The model under review builds one solid part; all positions refer to its coordinate system, in mm. Face numbers are marked on the shaded views. A direction names the side the tool comes from. Round coordinates to 2 decimals unless told otherwise and drop trailing zeros. Order: outer loops, then holes, each group sorted by start corner. A loop starts at its lowest first (then second) coordinate and runs counter-clockwise, first axis right, second up. Notation, with made-up numbers: M 39.5,-10 L 58.5,-10 A10 cw 58.5,3 Z; hole C 36,52.5 d7. An arc over 180 degrees is marked long. Answer as a JSON object with one key per item and string values. Group by question number.
1) Consider section A-A, the plane y = 19. Write out the cut boundary in (x, z).
2) Insertion check: pin 1 Ø2 at (y, z) = (11.5, -5.5) entering from +X; pin 2 Ø3 at (x, z) = (36.75, -17.5) entering from +Y. Each pin has a flat end and moves straight along its axis. Give the tip position at first contact, or say it passes through.
3) To check wall thickness, follow line 1 (X direction, y = 1.4, z = -17.5); line 2 (X direction, y = 8, z = -12); line 3 (Y direction, x = 44.45, z = -30). State the ranges of each line that lie inside material, in increasing order.
4) For the marked faces 4 and 5, list the 3-axis set-ups (+Z, -Z, +X, -X, +Y, -Y) from which the entire face can be reached by the end or side of a thin tool; tool diameter is ignored.
5) The part is to be moulded in two halves that separate along X. For the marked faces 1, 2 and 3, say which applies: +X half, -X half, draft (parallel to the pull), parting line (faces both ways), or undercut.
6) Consider section D-D, the plane z = -17.5. Write out the cut boundary in (x, y).
7) Consider section C-C, the plane x = 9.25. Write out the cut boundary in (y, z), then the cut area to 3 significant figures.
8) Consider section B-B, the plane z = -21.5. Write out the cut boundary in (x, y).
Autodesk Inventor part; units mm, degrees
ref_plane "YZ Plane" through (0, 0, 0) normal (1, 0, 0) x (0, 1, 0)
ref_plane "XZ Plane" through (0, 0, 0) normal (0, 1, 0) x (-1, 0, 0)
ref_plane "XY Plane" through (0, 0, 0) normal (0, 0, 1) x (1, 0, 0)
sketch "Boceto1" plane through (0, 0, 0) normal (0, 0, 1) x (1, 0, 0)
  line L0 (0, 0) -> (46, 0)
  line L1 (46, 0) -> (46, 21)
  line L2 (46, 21) -> (43, 21)
  line L3 (43, 21) -> (43, 3)
  line L4 (43, 3) -> (3, 3)
  line L5 (3, 3) -> (3, 21)
  line L6 (3, 21) -> (0, 21)
  line L7 (0, 21) -> (0, 0)
extrude "Extrusión1" add sketch "Boceto1" against normal blind 35
sketch "Boceto2" plane through (46, 0, 0) normal (1, 0, 0) x (0, 0, -1)
  circle A0 centre (5, 12) radius 2.5
  circle A1 centre (30, 12) radius 2.5
extrude "Extrusión2" cut sketch "Boceto2" against normal blind 60 contours A0
extrude "Extrusión3" cut sketch "Boceto2" against normal blind 60 contours A1
fillet "Empalme1" radius 5 4 edges at (1.5, 21, 0) (1.5, 21, -35) (44.5, 21, 0) (44.5, 21, -35)
sketch "Boceto3" plane through (3, 3, 0) normal (0, 1, 0) x (1, 0, 0)
  line L0 (8.75, 23.5) -> (31.25, 23.5)
  line L1 (31.25, 23.5) -> (31.25, 11.5)
  line L2 (31.25, 11.5) -> (8.75, 11.5)
  line L3 (8.75, 11.5) -> (8.75, 23.5)
  line L4 (8.75, 23.5) -> (8.75, 17.5)
  circle A0 centre (6.25, 17.5) radius 1.25
  line L5 (31.25, 23.5) -> (31.25, 17.5)
  circle A1 centre (33.75, 17.5) radius 1.25
  point P0 (-3, 0)
  point P1 (0, 35)
extrude "Extrusión4" cut sketch "Boceto3" against normal blind 60 contours L0 L1 L2 L3
extrude "Extrusión5" cut sketch "Boceto3" against normal blind 60 contours A0 | A1
properties part number "8_1"
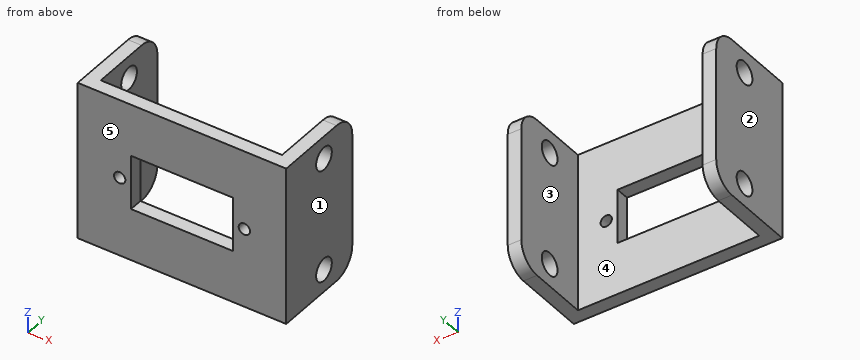
Results list:
{
 "1": {"outline": "M 0,-34 L 3,-34 L 3,-1 L 0,-1 Z; M 43,-34 L 46,-34 L 46,-1 L 43,-1 Z"},
 "2": {"pin 1": "through", "pin 2": "y = 3"},
 "3": {"line 1": "0 to 8, 10.5 to 11.75, 34.25 to 35.5, 38 to 46", "line 2": "0 to 3, 43 to 46", "line 3": "0 to 9.5, 14.5 to 21"},
 "4": {"face 4": "+Z, -Z, +Y", "face 5": "+Z, -Z, +X, -X, -Y"},
 "5": {"face 1": "+X half", "face 2": "-X half", "face 3": "undercut"},
 "6": {"outline": "M 0,0 L 8,0 L 8,3 L 3,3 L 3,21 L 0,21 Z; M 10.5,0 L 11.75,0 L 11.75,3 L 10.5,3 Z; M 34.25,0 L 35.5,0 L 35.5,3 L 34.25,3 Z; M 38,0 L 46,0 L 46,21 L 43,21 L 43,3 L 38,3 Z"},
 "7": {"outline": "M 0,-35 L 3,-35 L 3,-18.75 L 0,-18.75 Z; M 0,-16.25 L 3,-16.25 L 3,0 L 0,0 Z", "area": "97.5 mm^2"},
 "8": {"outline": "M 0,0 L 11.75,0 L 11.75,3 L 3,3 L 3,21 L 0,21 Z; M 34.25,0 L 46,0 L 46,21 L 43,21 L 43,3 L 34.25,3 Z"}
}
